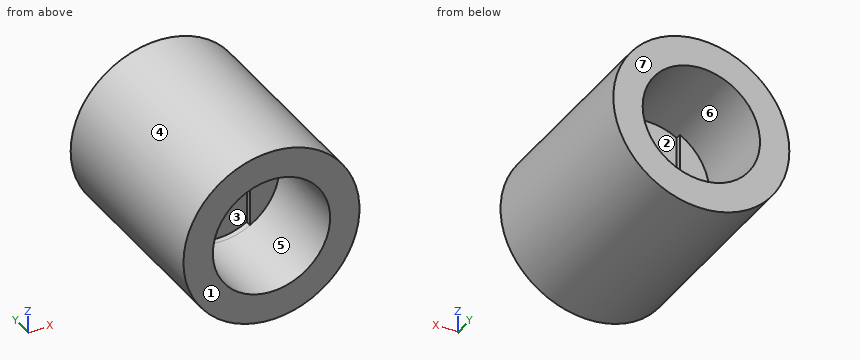
Autodesk Inventor part; units mm, degrees
ref_plane "YZ Plane" through (0, 0, 0) normal (1, 0, 0) x (0, 1, 0)
ref_plane "XZ Plane" through (0, 0, 0) normal (0, 1, 0) x (-1, 0, 0)
ref_plane "XY Plane" through (0, 0, 0) normal (0, 0, 1) x (1, 0, 0)
sketch "Sketch1" plane through (0, 0, 0) normal (0, 1, 0) x (-1, 0, 0)
  circle A0 centre (0, 0) radius 3
  circle A1 centre (0, 0) radius 2
  dimension "d0" = 6
  dimension "d3" = 4
extrude "Extrusion1" add sketch "Sketch1" along normal blind 6.9 contours A0 | A1
extrude "Extrusion2" cut sketch "Sketch1" along normal blind 3.1 contours A1
sketch "Sketch2" plane through (0, 6.9, 0) normal (0, 1, 0) x (1, 0, 0)
  circle A0 centre (0, 0) radius 2
extrude "Extrusion3" cut sketch "Sketch2" against normal blind 3.1
sketch "Sketch3" plane through (0, 3.8, 0) normal (0, 1, 0) x (1, 0, 0)
  line L0 (1, 2) -> (-1, 2)
  line L1 (-1, 2) -> (-1, -2)
  line L2 (-1, -2) -> (1, -2)
  line L3 (1, -2) -> (1, 2)
  line L4 (1, 2) -> (-1, -2) construction
  line L5 (-1, 2) -> (1, -2) construction
  circle A0 centre (0, 0) radius 2
  point P0 (1, -1.7321)
  point P1 (1, 1.7321)
  point P2 (-1, 1.7321)
  point P3 (-1, -1.7321)
  dimension "d8" = 2
extrude "Extrusion4" cut sketch "Sketch3" against normal blind 0.2 contours A0 L3 L1
sketch "Sketch4" plane through (0, 3.1, 0) normal (0, -1, 0) x (1, 0, 0)
  line L0 (1, -1.7321) -> (1, 1.7321)
  arc A0 (-1, -1.7321) -> (1, -1.7321) centre (0, 0) ccw
  line L1 (-1, 1.7321) -> (-1, -1.7321)
  arc A1 (1, 1.7321) -> (-1, 1.7321) centre (0, 0) ccw
extrude "Extrusion5" cut sketch "Sketch4" against normal blind 0.2
properties part number "Printed Standoff 6.9mm"
Geometry: final body of the model. Coordinates: model frame, mm. Face numbers are marked on the shaded views. A direction names the side the tool comes from. Give positions to 0.01 mm unless a question says otherwise; leave off trailing zeros. Order: outer loops, then holes, each group sorted by start corner. A loop starts at its lowest first (then second) coordinate and runs counter-clockwise, first axis right, second up. Notation, with made-up numbers: (-17.5, -6.5) - (29.5, -6.5) arc R37 ccw to (29.5, 29.5) - close; hole circle Ø8 at (-16, -10). An arc over 180 degrees is marked (long way). Use CSV: the item, a comma, the result in double quotes.
1. Access query for the marked faces 5, 6 and 7. Directions: +Z, -Z, +X, -X, +Y, -Y. A direction counts if a zero-diameter tool reaches every point of the face in a straight line with its end or side. Return the directions, or none.
Answers below:
face 5,"-Y"
face 6,"+Y"
face 7,"+Z, -Z, +X, -X, +Y"
2. Contact query for flat-ended pins moving along their axis: pin 1 (2 mm diameter, centred on x = 0.5, z = -0.5, fed in from +Y); pin 2 (0.8 mm diameter, centred on x = 1.5, z = 0, fed in from -Y); pin 3 (0.6 mm diameter, centred on x = 0, z = -1, fed in from -Y). Output: stop coordinate, or through.
Answers below:
pin 1,"y = 3.8"
pin 2,"y = 3.1"
pin 3,"y = 3.3"
3. Section query B-B (y = 5). Output: boundary loops of the cut face in (x, z), plus the area to 3 significant figures.
Answers below:
outline,"circle Ø6 at (0, 0); hole circle Ø4 at (0, 0)"
area,"15.7 mm2"
4. Section query A-A (z = 0). Output: boundary loops of the cut face in (x, y).
Answers below:
outline,"(-3, 0) - (-2, 0) - (-2, 3.1) - (-1, 3.1) - (-1, 3.3) - (1, 3.3) - (1, 3.1) - (2, 3.1) - (2, 0) - (3, 0) - (3, 6.9) - (2, 6.9) - (2, 3.8) - (1, 3.8) - (1, 3.6) - (-1, 3.6) - (-1, 3.8) - (-2, 3.8) - (-2, 6.9) - (-3, 6.9) - close"
5. Section query D-D (y = 3.5). Output: boundary loops of the cut face in (x, z).
Answers below:
outline,"circle Ø6 at (0, 0)"
6. Material intervals for line 1 along Z through (x, y) = (0, 1.1); line 2 along Y through (x, z) = (0.8, 1.75), sorted ascending. Write a range as from..to.
Answers below:
line 1,"-3..-2, 2..3"
line 2,"3.3..3.6"
7. Mould query, pull axis Z, two halves, no side actions, for the marked faces 1, 2, 3 and 4. Classes: +Z half, -Z half, draft (parallel to the pull), parting line (faces both ways), or undercut.
Answers below:
face 1,"draft"
face 2,"undercut"
face 3,"undercut"
face 4,"parting line"
